Part model, mm, in its own coordinate system. A direction names the side the tool comes from. Coordinates: 2 decimals unless noted, no trailing zeros. Write each loop counter-clockwise with the first axis right and the second up, starting at its lowest first coordinate (ties: lowest second). Pieces come first, ordered by that corner, then holes. Notation, with made-up numbers: (-29, 81) - (-5, 81) arc R18 cw to (-5, 93) - close; hole circle Ø3 at (0.5, 17.5). An arc over 180 degrees is marked (long way). Use a Markdown table: item, result.
```python
from build123d import *

# Parameters (mm, degrees)
SKETCH_1_R          = 4.1
SKETCH_1_R_2        = 1.5
EXTRUDE_1_DEPTH     = 10
SKETCH_2_W          = 10.2
SKETCH_2_H          = 10.2
CUT_EXTRUDE_1_DEPTH = 5
EXTRUDE_2_DEPTH     = 10


with BuildPart() as part:
    # ｽｹｯﾁ1 → ﾎﾞｽ - 押し出し1 (new body)
    with BuildSketch(Plane(origin=(0, 0, 0), x_dir=(1, 0, 0), z_dir=(0, 1, 0))):
        with BuildLine():
            Line((-90.755581693, -47.201953746), (29.244418307, -19.748139436))
            ThreePointArc((29.244418307, -19.748139436), (34.834131004, -16.232897902), (37.014221558, -10))
            Line((37.014221558, -10), (37.014221558, 10))
            ThreePointArc((37.014221558, 10), (34.834131004, 16.232897902), (29.244418307, 19.748139436))
            Line((29.244418307, 19.748139436), (-90.755581693, 47.201953746))
            ThreePointArc((-90.755581693, 47.201953746), (-99.218676344, 45.273723756), (-102.985778442, 37.45381431))
            Line((-102.985778442, 37.45381431), (-102.985778442, -37.45381431))
            ThreePointArc((-102.985778442, -37.45381431), (-99.218676344, -45.273723756), (-90.755581693, -47.201953746))
        make_face()
        with Locations(Location((-82.985778442, 0, 0), (0, 0, 270))):
            Circle(SKETCH_1_R, mode=Mode.SUBTRACT)
        with Locations(Location((27.014221558, 0, 0), (0, 0, 270))):
            Circle(SKETCH_1_R, mode=Mode.SUBTRACT)
        with Locations(Location((-87.985778442, 35, 0), (0, 0, 270))):
            Circle(SKETCH_1_R_2, mode=Mode.SUBTRACT)
        with Locations(Location((-87.985778442, -35, 0), (0, 0, 270))):
            Circle(SKETCH_1_R_2, mode=Mode.SUBTRACT)
    extrude(amount=EXTRUDE_1_DEPTH)

    # ｽｹｯﾁ2 → ｶｯﾄ - 押し出し1 (cut)
    with BuildSketch(Plane.XZ):
        with Locations((-87.985778442, 35)):
            Rectangle(SKETCH_2_W, SKETCH_2_H)
        with Locations((-87.985778442, -35)):
            Rectangle(SKETCH_2_W, SKETCH_2_H)
    extrude(amount=-CUT_EXTRUDE_1_DEPTH, mode=Mode.SUBTRACT)

    # ｽｹｯﾁ3 → ﾎﾞｽ - 押し出し2 (add)
    with BuildSketch(Plane.XZ):
        Polygon((-46.56667029, 37.092335677), (-36.818530855, 34.862138928), (-39.048727604, 25.113999492), (-48.79686704, 27.344196242), align=None)
        Polygon((-46.56667029, -37.092335677), (-36.818530855, -34.862138928), (-39.048727604, -25.113999492), (-48.79686704, -27.344196242), align=None)
    extrude(amount=EXTRUDE_2_DEPTH)


solid = part.part
```
Item 1: Which spindle directions (+Z, -Z, +X, -X, +Y, -Y) get a long thin tool onto all of the face, cutting with end or side? Do faces 4 (the face through (-82.886, 2, -35)), 5 (the face through (-43.855, -4.93, 26.213)), 6 (the face through (-88.9, 7.46, 33.81)). Say none if no direction does.
From the geometry:
| item | result |
|---|---|
| face 4 | -Y |
| face 5 | -X, -Y |
| face 6 | +Y, -Y |
Item 2: Drop flat-ended pins along their axis: P1, Ø5.5, axis at x = -87, y = 3.5, coming from the +Z side; P2, Ø12, axis at x = 10, y = 6.5, coming from the +Z side; P3, Ø6, axis at x = -86.5, y = 3.5, coming from the -Z side; P4, Ø2.5, axis at x = -87.99, z = -35, coming from the -Y side. Give the stop position or say it passes through.
From the geometry:
| item | result |
|---|---|
| P1 | z = 46.97 |
| P2 | z = 25.52 |
| P3 | z = -46.91 |
| P4 | through |
Item 3: Drill centre lines: probe 1 along X at (y, z) = (2, 0); probe 2 along Y at (x, z) = (-69.5, -24); probe 3 along X at (y, z) = (1.25, -3). Where is each one in solid material? Low to high.
From the geometry:
| item | result |
|---|---|
| probe 1 | -102.99 to -87.09, -78.89 to 22.91, 31.11 to 37.01 |
| probe 2 | 0 to 10 |
| probe 3 | -102.99 to -85.78, -80.19 to 24.22, 29.81 to 37.01 |
Item 4: Band-saw the part on D-D, the plane y = 8.5. Give the cut face in (x, z).
From the geometry:
| item | result |
|---|---|
| outline | (-102.99, -37.45) arc R10 ccw to (-90.76, -47.2) - (29.24, -19.75) arc R10 ccw to (37.01, -10) - (37.01, 10) arc R10 ccw to (29.24, 19.75) - (-90.76, 47.2) arc R10 ccw to (-102.99, 37.45) - close; hole circle Ø3 at (-87.99, -35); hole circle Ø3 at (-87.99, 35); hole circle Ø8.2 at (-82.99, 0); hole circle Ø8.2 at (27.01, 0) |
Item 5: Band-saw the part on C-C, the plane x = -64. Give the cut face in (y, z), then the cut area to 3 significant figures.
From the geometry:
| item | result |
|---|---|
| outline | (0, -41.08) - (10, -41.08) - (10, 41.08) - (0, 41.08) - close |
| area | 822 mm^2 |
Item 6: Two-plate mould, pull along Z, no slides. Class faces 1 (the face through (34.89, 4.93, -16.16)), 2 (the face through (-50, 10, -1)), 3 (the face through (31.08, 4.93, -0.53)): pulls with the +Z half, pulls with the -Z half, needs draft (parallel to the pull), parting line crosses it, or undercut.
From the geometry:
| item | result |
|---|---|
| face 1 | pulls with the -Z half |
| face 2 | needs draft |
| face 3 | undercut |
Item 7: Band-saw the part on B-B, the plane y = 1.75. Give the cut face in (x, z), then the cut area to 3 significant figures.
From the geometry:
| item | result |
|---|---|
| outline | (-102.99, -37.45) arc R10 ccw to (-90.76, -47.2) - (29.24, -19.75) arc R10 ccw to (37.01, -10) - (37.01, 10) arc R10 ccw to (29.24, 19.75) - (-90.76, 47.2) arc R10 ccw to (-102.99, 37.45) - close; hole (-93.09, -40.1) - (-82.89, -40.1) - (-82.89, -29.9) - (-93.09, -29.9) - close; hole (-93.09, 29.9) - (-82.89, 29.9) - (-82.89, 40.1) - (-93.09, 40.1) - close; hole circle Ø8.2 at (-82.99, 0); hole circle Ø8.2 at (27.01, 0) |
| area | 9,110 mm^2 |
Item 8: Band-saw the part on A-A, the plane z = 0. Give the cut face in (x, y), then the cut area to 3 significant figures.
From the geometry:
| item | result |
|---|---|
| outline | (-102.99, 0) - (-87.09, 0) - (-87.09, 10) - (-102.99, 10) - close; (-78.89, 0) - (22.91, 0) - (22.91, 10) - (-78.89, 10) - close; (31.11, 0) - (37.01, 0) - (37.01, 10) - (31.11, 10) - close |
| area | 1,240 mm^2 |
